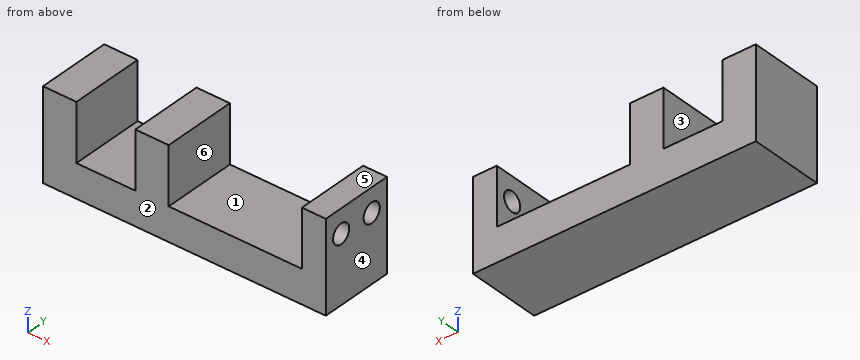
from build123d import *

# Parameters (mm, degrees)
F0_W     = 7
F0_H     = 15.5
F0_W_2   = 12.34
F0_W_3   = 27.91
F0_W_4   = 5
F1_DEPTH = 7
F2_DEPTH = 19
F4_DEPTH = 25


with BuildPart() as f1:
    # F0 (on Top) → F1 (new body)
    with BuildSketch(Plane.XY):
        with Locations((-86.9522068564, 0)):
            Rectangle(F0_W, F0_H)
        with Locations((-77.2822068564, 0)):
            Rectangle(F0_W_2, F0_H)
        with Locations((-67.6122068564, 0)):
            Rectangle(F0_W, F0_H)
        with Locations((-50.1572068564, 0)):
            Rectangle(F0_W_3, F0_H)
        with Locations((-33.7022068564, 0)):
            Rectangle(F0_W_4, F0_H)
    extrude(amount=F1_DEPTH)

    # F0 (on Top) → F2 (join)
    with BuildSketch(Plane.XY):
        with Locations((-86.9522068564, 0)):
            Rectangle(F0_W, F0_H)
        with Locations((-67.6122068564, 0)):
            Rectangle(F0_W, F0_H)
        with Locations((-33.7022068564, 0)):
            Rectangle(F0_W_4, F0_H)
    extrude(amount=F2_DEPTH)

    # F3 (on face) → F4 (cut)
    with BuildSketch(Plane.YZ.offset(-31.2022068564)):
        with BuildLine():
            Line((-5.925, 14), (-1.825, 14))
            ThreePointArc((-1.825, 14), (-3.875, 16.05), (-5.925, 14))
        make_face()
        with BuildLine():
            ThreePointArc((5.925, 14), (3.875, 16.05), (1.825, 14))
            Line((1.825, 14), (5.925, 14))
        make_face()
        with BuildLine():
            Line((5.925, 14), (1.825, 14))
            ThreePointArc((1.825, 14), (3.875, 11.95), (5.925, 14))
        make_face()
        with BuildLine():
            ThreePointArc((-5.925, 14), (-3.875, 11.95), (-1.825, 14))
            Line((-1.825, 14), (-5.925, 14))
        make_face()
    extrude(amount=-F4_DEPTH, mode=Mode.SUBTRACT)


solid = f1.part
Read the model definition and answer for the solid it produces. Units are mm, in the model's axes. Face numbers are marked on the shaded views. A direction names the side the tool comes from. Round coordinates to 2 decimals unless told otherwise and drop trailing zeros. Order: outer loops, then holes, each group sorted by start corner. A loop starts at its lowest first (then second) coordinate and runs counter-clockwise, first axis right, second up. Notation, with made-up numbers: (81.25, 54.5) - (98.25, 54.5) arc R6 cw to (98.25, 62.5) - close; hole circle Ø1 at (4.25, 11). An arc over 180 degrees is marked (long way). Use one line per item in the form item = value. Start each with the question number.
(1) Find the intervals of material crossed by line 1 along X through (y, z) = (-2.5, 8.25); line 2 along Y through (x, z) = (-32.4, 14) (3 decimals); line 3 along X through (y, z) = (-3.25, 15), in increasing order. Write a range as from..to.
(2) Determine the mould class of the marked faces 3, 4, 5 and 6 for opening direction X: +X half, -X half, draft (parallel to the pull), parting line (faces both ways), or undercut.
(3) The part is cut by section B-B (y = 4.25). Give the vertices of the cut face in (x, z), then the cut area to 3 significant figures.
(4) The part is cut by section A-A (z = 14). Give the vertices of the cut face in (x, y) (3 decimals).
(5) The part is cut by section C-C (x = -80). Give the vertices of the cut face in (y, z), then the cut area to 4 significant figures.
(6) Flat-ended cylindrical pins translate along their axes: pin 1 Ø3.5 at (x, y) = (-76, 0.5) entering from +Z; pin 2 Ø3.5 at (y, z) = (-3.875, 14) entering from +X; pin 3 Ø1.5 at (x, y) = (-52, 2.5) entering from -Z. Find the tip coordinate at first contact, or state that the pin passes through.
(7) For the marked faces 1 and 2, determine the directions among +Z, -Z, +X, -X, +Y, -Y from which every point of the face is accessible in a straight line to the end or side of a thin tool.
Checked values:
q1.line_1 = -90.45..-83.45, -71.11..-64.11, -36.2..-31.2
q1.line_2 = -7.75..-5.925, -1.825..1.825, 5.925..7.75
q1.line_3 = -90.45..-83.45, -71.11..-64.11
q2.face_3 = undercut
q2.face_4 = +X half
q2.face_5 = draft
q2.face_6 = undercut
q3.outline = (-90.45, 0) - (-31.2, 0) - (-31.2, 11.98) - (-36.2, 11.98) - (-36.2, 7) - (-64.11, 7) - (-64.11, 19) - (-71.11, 19) - (-71.11, 7) - (-83.45, 7) - (-83.45, 19) - (-90.45, 19) - close; (-36.2, 16.02) - (-31.2, 16.02) - (-31.2, 19) - (-36.2, 19) - close
q3.area = 623 mm^2
q4.outline = (-90.452, -7.75) - (-83.452, -7.75) - (-83.452, 7.75) - (-90.452, 7.75) - close; (-71.112, -7.75) - (-64.112, -7.75) - (-64.112, 7.75) - (-71.112, 7.75) - close; (-36.202, -7.75) - (-31.202, -7.75) - (-31.202, -5.925) - (-36.202, -5.925) - close; (-36.202, -1.825) - (-31.202, -1.825) - (-31.202, 1.825) - (-36.202, 1.825) - close; (-36.202, 5.925) - (-31.202, 5.925) - (-31.202, 7.75) - (-36.202, 7.75) - close
q5.outline = (-7.75, 0) - (7.75, 0) - (7.75, 7) - (-7.75, 7) - close
q5.area = 108.5 mm^2
q6.pin_1 = 7
q6.pin_2 = -64.11
q6.pin_3 = 0
q7.face_1 = +Z, +Y, -Y
q7.face_2 = +Z, -Z, +X, -X, -Y
